Part print with two shaded views. Sizes in mm from the minimum x, y, z corner. Coordinates: 2 decimals unless noted, no trailing zeros. Order: outer loops, then holes, each group sorted by start corner. A loop starts at its lowest first (then second) coordinate and runs counter-clockwise, first axis right, second up. Notation, with made-up numbers: (46, 26) - (72, 26) arc R31 cw to (72, 50) - close; hole circle Ø7 at (-29.5, 9). An arc over 180 degrees is marked (long way). One line per item, written item: value.
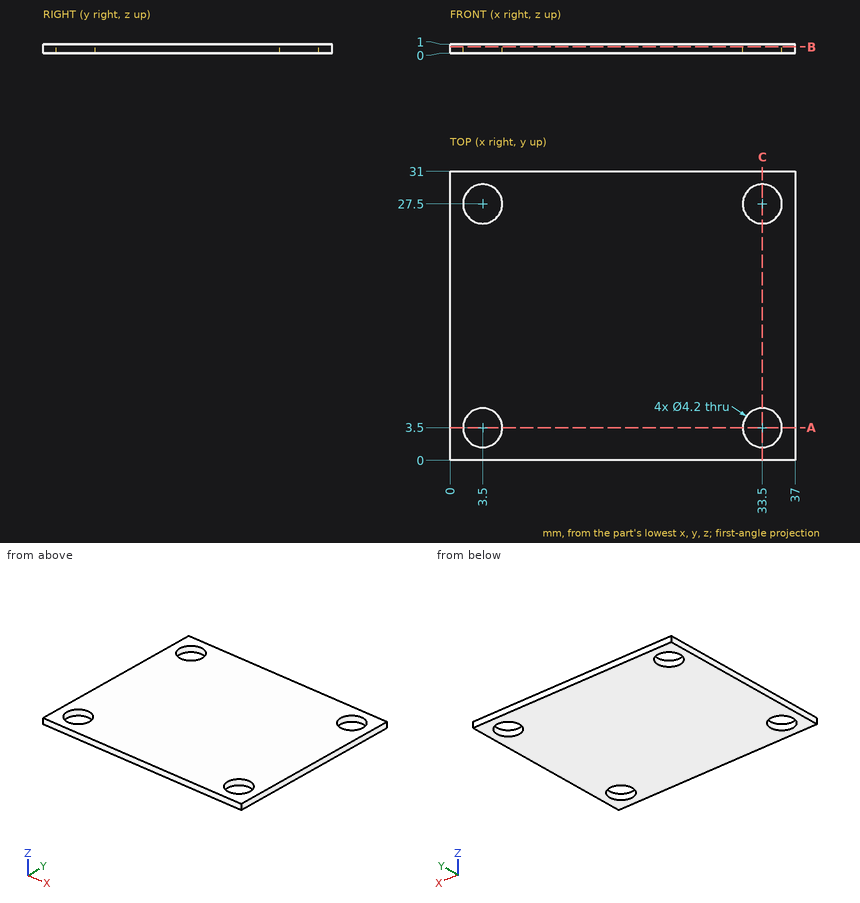
1. Band-saw the part on C-C, the plane x = 33.5. Give the cut face in (y, z), and give its area (3 significant figures).
Values found:
outline: (0, 0) - (1.4, 0) - (1.4, 1) - (0, 1) - close; (5.6, 0) - (25.4, 0) - (25.4, 1) - (5.6, 1) - close; (29.6, 0) - (31, 0) - (31, 1) - (29.6, 1) - close
area: 22.6 mm2
2. Band-saw the part on B-B, the plane z = 0.7. Give the cut face in (x, y), and give its area (3 significant figures).
Values found:
outline: (0, 0) - (37, 0) - (37, 31) - (0, 31) - close; hole circle Ø4.2 at (3.5, 3.5); hole circle Ø4.2 at (3.5, 27.5); hole circle Ø4.2 at (33.5, 3.5); hole circle Ø4.2 at (33.5, 27.5)
area: 1,090 mm2
3. Band-saw the part on A-A, the plane y = 3.5. Give the cut face in (x, z), and give its area (3 significant figures).
Values found:
outline: (0, 0) - (1.4, 0) - (1.4, 1) - (0, 1) - close; (5.6, 0) - (31.4, 0) - (31.4, 1) - (5.6, 1) - close; (35.6, 0) - (37, 0) - (37, 1) - (35.6, 1) - close
area: 28.6 mm2
4. Probe line 1 along X through (y, z) = (27.5, 0.3); line 2 along Y through (x, z) = (33.5, 0.75); line 3 along Y through (x, z) = (2, 0.6). List the from-to ranges inside material, lowest first.
Values found:
line 1: x = 0 to 1.4, 5.6 to 31.4, 35.6 to 37
line 2: y = 0 to 1.4, 5.6 to 25.4, 29.6 to 31
line 3: y = 0 to 2.03, 4.97 to 26.03, 28.97 to 31
5. Flat gauge pins, fed straight in: P1, Ø5.5, axis at x = 33.5, y = 27.5, coming from the +Z side; P2, Ø4, axis at x = 3.5, y = 3.5, coming from the -Z side. Where does each tip first touch, or does it go through?
Values found:
P1: stops at z = 1
P2: passes through
